Can you work these out from the model? Positions are in its coordinate system, mm. Face numbers are marked on the shaded views. A direction names the side the tool comes from. Give positions to 0.01 mm unless a question says otherwise; leave off trailing zeros. Order: outer loops, then holes, each group sorted by start corner. A loop starts at its lowest first (then second) coordinate and runs counter-clockwise, first axis right, second up.
Item 1: If we mould it in two halves opening along Y, with no side actions, what happens to the marked faces 5, 6, 7 and 8? For each: +Y half, -Y half, draft (parallel to the pull), parting line (faces both ways), or undercut.
Item 2: I'm going to push flat-ended pins straight in: pin 1 Ø1 at (x, z) = (28.5, -8) entering from +Y; pin 2 Ø4 at (x, z) = (32, -14.5) entering from +Y; pin 3 Ø2 at (y, z) = (-37, -26.5) entering from +X; pin 4 Ø4.5 at (x, y) = (-1, -51.5) entering from -Z. Where does each tip first touch, or does it pass through?
Item 3: If I drill on line 1 along Y through (x, z) = (0, -3.4) (3 decimals); line 2 along X through (y, z) = (0, -7.05) (3 decimals); line 3 along Z through (x, y) = (-19, 30.5), over which ranges is the centre line in solid material (lowest first)?
Item 4: Which directions (+Z, -Z, +X, -X, +Y, -Y) give clear straight access to the entire face, cutting with the end or side of a thin tool? Please do the marked faces 1, 2, 3 and 4.
Item 5: I want a section at B-B, the plane y = 0. Count the separate pieces of the cut face and the enclosed holes in it, then the cut area to 3 significant figures.
Item 6: I want a section at C-C, the plane z = -22. Write out the boundary of the cut face in (x, y), then the cut area to 3 significant figures.
Item 7: I want a section at A-A, the plane x = 59. Write out the boundary of the cut face in (y, z) (3 decimals), then the cut area to 3 significant figures.
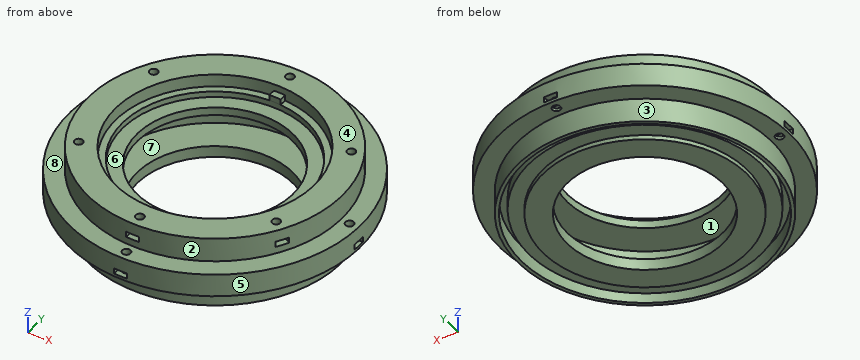
```python
from build123d import *

# Parameters (mm, degrees)
SKETCH2_R           = 1.8
CUT_EXTRUDE1_DEPTH  = 10
SKETCH3_W           = 5.6
SKETCH3_H           = 10.691433847
CUT_EXTRUDE2_DEPTH  = 2.4
BOSS_EXTRUDE1_DEPTH = 2.5
SKETCH5_R           = 1.8
CUT_EXTRUDE3_DEPTH  = 92.417862724
SKETCH6_W           = 5.6
SKETCH6_H           = 10.168713577
SKETCH6_W_2         = 10.168713577
SKETCH6_H_2         = 5.6
CUT_EXTRUDE4_DEPTH  = 2.4


with BuildPart() as part:
    # Sketch1 → Revolve1 (revolve)
    with BuildSketch(Plane(origin=(0, 0, 0), x_dir=(1, 0, 0), z_dir=(0, 1, 0))):
        Polygon((43.05, 0), (43.05, 5.5), (40.025, 5.5), (40.025, 8.05), (33.75, 8.05), (33.75, 11.55), (47.68, 11.55), (47.68, 25.95), (33.75, 25.95), (33.75, 30.95), (44.2, 30.95), (44.2, 28.95), (50.35, 28.95), (50.35, 23.95), (53.5, 23.95), (53.5, 30.95), (55, 30.95), (55, 20.475), (63, 20.475), (63, 10.475), (55, 10.475), (55, 0), align=None)
    revolve(axis=Axis((0, 0, 39.851832449), (0, 0, -1)))

    # Sketch2 → Cut-Extrude1 (cut)
    with BuildSketch(Plane.XY):
        with Locations((0, 50)):
            Circle(SKETCH2_R)
        with Locations((43.301270189, 25)):
            Circle(SKETCH2_R)
        with Locations((43.301270189, -25)):
            Circle(SKETCH2_R)
        with Locations((0, -50)):
            Circle(SKETCH2_R)
        with Locations((-43.301270189, -25)):
            Circle(SKETCH2_R)
        with Locations((-43.301270189, 25)):
            Circle(SKETCH2_R)
    extrude(amount=-CUT_EXTRUDE1_DEPTH, mode=Mode.SUBTRACT)

    # Sketch3 → Cut-Extrude2 (cut)
    with BuildSketch(Plane.XY.offset(-5)):
        with Locations((0, 52.545716924)):
            Rectangle(SKETCH3_W, SKETCH3_H)
        Polygon((51.535452373, 26.520845793), (48.735452373, 31.370588054), (39.476399059, 26.024871131), (42.276399059, 21.175128869), align=None)
        Polygon((48.735452373, -31.370588054), (51.535452373, -26.520845793), (42.276399059, -21.175128869), (39.476399059, -26.024871131), align=None)
        with Locations((0, -52.545716924)):
            Rectangle(SKETCH3_W, SKETCH3_H)
        Polygon((-51.535452373, -26.520845793), (-48.735452373, -31.370588054), (-39.476399059, -26.024871131), (-42.276399059, -21.175128869), align=None)
        Polygon((-48.735452373, 31.370588054), (-51.535452373, 26.520845793), (-42.276399059, 21.175128869), (-39.476399059, 26.024871131), align=None)
    extrude(amount=-CUT_EXTRUDE2_DEPTH, mode=Mode.SUBTRACT)

    # Sketch4 → Boss-Extrude1 (add)
    with BuildSketch(Plane.XY.offset(-5.5)):
        with BuildLine():
            Line((-2.45, 42.980228012), (-2.45, 39.949945244))
            ThreePointArc((-2.45, 39.949945244), (0, 40.025), (2.45, 39.949945244))
            Line((2.45, 39.949945244), (2.45, 42.980228012))
            ThreePointArc((2.45, 42.980228012), (0, 43.05), (-2.45, 42.980228012))
        make_face()
    extrude(amount=BOSS_EXTRUDE1_DEPTH)

    # Sketch5 → Cut-Extrude3 (cut, through all)
    with BuildSketch(Plane.XY.offset(-10.475)):
        with Locations((0, 59)):
            Circle(SKETCH5_R)
        with Locations((59, 0)):
            Circle(SKETCH5_R)
        with Locations((0, -59)):
            Circle(SKETCH5_R)
        with Locations((-59, 0)):
            Circle(SKETCH5_R)
    extrude(amount=-CUT_EXTRUDE3_DEPTH, mode=Mode.SUBTRACT)

    # Sketch6 → Cut-Extrude4 (cut)
    with BuildSketch(Plane.XY.offset(-16.775)):
        with Locations((0, 61.284356789)):
            Rectangle(SKETCH6_W, SKETCH6_H)
        with Locations((61.284356789, 0)):
            Rectangle(SKETCH6_W_2, SKETCH6_H_2)
        with Locations((0, -61.284356789)):
            Rectangle(SKETCH6_W, SKETCH6_H)
        with Locations((-61.284356789, 0)):
            Rectangle(SKETCH6_W_2, SKETCH6_H_2)
    extrude(amount=-CUT_EXTRUDE4_DEPTH, mode=Mode.SUBTRACT)


solid = part.part
```
Results list:
1. face 5: parting line
1. face 6: undercut
1. face 7: undercut
1. face 8: draft
2. pin 1: stops at y = 47.34
2. pin 2: stops at y = 55.4
2. pin 3: stops at x = 41.58
2. pin 4: stops at z = -30.95
3. line 1: y = -55 to -51.8, -48.2 to -43.05, 40.025 to 48.2, 51.8 to 55
3. line 2: x = -55 to -40.025, 40.025 to 55
3. line 3: z = -30.95 to -25.95, -11.55 to -8.05
4. face 1: none
4. face 2: +Z
4. face 3: -Z
4. face 4: +Z, +X, -X, +Y, -Y
5. separate pieces: 6
5. enclosed holes: 0
5. area: 784 mm2
6. outline: circle Ø110 at (0, 0); hole circle Ø95.36 at (0, 0)
6. area: 2,360 mm2
7. outline: (-22.091, -20.475) - (-1.8, -20.475) - (-1.8, -19.175) - (-2.8, -19.175) - (-2.8, -16.775) - (-1.8, -16.775) - (-1.8, -10.475) - (-22.091, -10.475) - close; (1.8, -20.475) - (22.091, -20.475) - (22.091, -10.475) - (1.8, -10.475) - (1.8, -16.775) - (2.8, -16.775) - (2.8, -19.175) - (1.8, -19.175) - close
7. area: 401 mm2
